Read the model definition and answer for the solid it produces. Units are mm, in the model's axes. Coordinates: 2 decimals unless noted, no trailing zeros. Put each result on its own line as item: value.
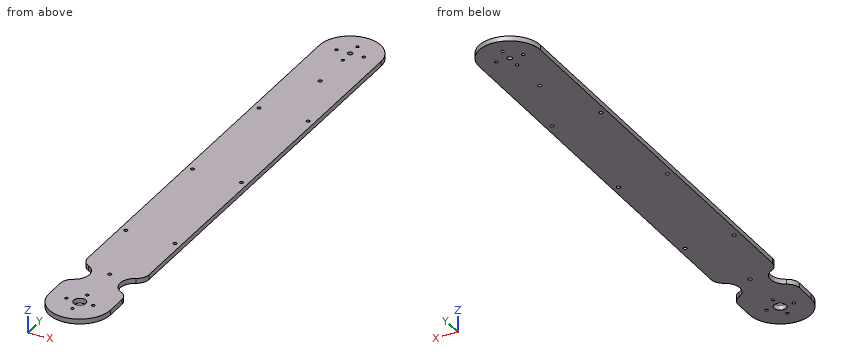
from build123d import *

# Parameters (mm, degrees)
SKETCH001_R             = 2
SKETCH001_R_2           = 1.25
SKETCH001_R_3           = 1.5
SKETCH001_R_4           = 5
PAD001_DEPTH            = 4
SKETCH002_R             = 12.5
POCKET_DEPTH            = 11
FILLET_R                = 10
BODY001_PLACEMENT_ANGLE = 180


with BuildPart() as part:
    # Sketch001 → Pad001 (new body)
    with BuildSketch(Plane.XY):
        with BuildLine():
            ThreePointArc((-25, 0), (0, -25), (25, 0))
            Line((25, 0), (25, 406.000606))
            ThreePointArc((25, 406.000606), (0, 431.000606), (-25, 406.000606))
            Line((-25, 0), (-25, 406.000606))
        make_face()
        with Locations((0, 0.000303)):
            Circle(SKETCH001_R, mode=Mode.SUBTRACT)
        with Locations((10.999698, 0.000303)):
            Circle(SKETCH001_R_2, mode=Mode.SUBTRACT)
        with Locations((0, 11)):
            Circle(SKETCH001_R_2, mode=Mode.SUBTRACT)
        with Locations((-10.999697, 0.000303)):
            Circle(SKETCH001_R_2, mode=Mode.SUBTRACT)
        with Locations((0, -10.999395)):
            Circle(SKETCH001_R_2, mode=Mode.SUBTRACT)
        with Locations((-20, 300.000454)):
            Circle(SKETCH001_R_3, mode=Mode.SUBTRACT)
        with Locations((20, 300.000454)):
            Circle(SKETCH001_R_3, mode=Mode.SUBTRACT)
        with Locations((-20, 200.000303)):
            Circle(SKETCH001_R_3, mode=Mode.SUBTRACT)
        with Locations((20, 200.000303)):
            Circle(SKETCH001_R_3, mode=Mode.SUBTRACT)
        with Locations((-20, 100.000152)):
            Circle(SKETCH001_R_3, mode=Mode.SUBTRACT)
        with Locations((20, 100.000152)):
            Circle(SKETCH001_R_3, mode=Mode.SUBTRACT)
        with Locations((0, 45)):
            Circle(SKETCH001_R_3, mode=Mode.SUBTRACT)
        with Locations((0, 406.000606)):
            Circle(SKETCH001_R_4, mode=Mode.SUBTRACT)
        with Locations((0, 417.000606)):
            Circle(SKETCH001_R_2, mode=Mode.SUBTRACT)
        with Locations((-10.999697, 406.000909)):
            Circle(SKETCH001_R_2, mode=Mode.SUBTRACT)
        with Locations((0, 395.001211)):
            Circle(SKETCH001_R_2, mode=Mode.SUBTRACT)
        with Locations((10.999698, 406.000909)):
            Circle(SKETCH001_R_2, mode=Mode.SUBTRACT)
        with Locations((0, 361.000606)):
            Circle(SKETCH001_R_3, mode=Mode.SUBTRACT)
    extrude(amount=PAD001_DEPTH)

    # Sketch002 (on Face24 of Pad001) → Pocket (cut)
    with BuildSketch(Plane.XY.offset(4)):
        with Locations((-25, 368.584032)):
            Circle(SKETCH002_R)
        with Locations((25, 368.584032)):
            Circle(SKETCH002_R)
    extrude(amount=-POCKET_DEPTH, mode=Mode.SUBTRACT)

    # Fillet
    fillet_edges = [part.edges().sort_by_distance(p)[0] for p in [
        (25, 381.084032, 2),
        (25, 356.084032, 2),
        (-25, 381.084032, 2),
        (-25, 356.084032, 2),
    ]]
    fillet(fillet_edges, radius=FILLET_R)


with BuildPart() as part_1:
    # Body001 placement: moved
    add(part.part.moved(Location((68.48, 410, 17.66))).rotate(Axis((68.48, 410, 17.66), (0, 0, 1)), BODY001_PLACEMENT_ANGLE))


solid = part_1.part
1) Straight lines are drawn through the part: line 1 (X direction, y = 365, z = 19.9); line 2 (Y direction, x = 58, z = 20.3); line 3 (Y direction, x = 65, z = 19.45). For each, find the intervals that lie inside material, in ascending order. Write a range as [from, to].
Answer list:
line 1: x = [43.48, 66.98], [69.98, 93.48]
line 2: y = [-18.7, 2.86], [5.14, 408.86], [411.14, 432.7]
line 3: y = [-20.76, 0.41], [7.59, 434.76]
2) Given pin 1 Ø1 at (x, z) = (61, 19) entering from -Y; pin 2 Ø2 at (x, z) = (85, 18) entering from -Y; pin 3 Ø2 at (x, z) = (50, 19) entering from -Y, each flat-ended and moving along its own axis, determine where each tip first touches the part or whether it passes through.
Answer list:
pin 1: stops at y = -20.01
pin 2: stops at y = -15.6
pin 3: stops at y = -13.87
3) Find section A-A, the plane z = 18.45. Count the separate pieces of the cut face and the enclosed holes in it, plus the area to 3 significant figures.
Answer list:
separate pieces: 1
enclosed holes: 18
area: 21,500 mm^2
